Geometry: final body of the model. Coordinates: model frame, mm. Face numbers are marked on the shaded views. A direction names the side the tool comes from. Coordinates: 2 decimals unless noted, no trailing zeros. Write each loop counter-clockwise with the first axis right and the second up, starting at its lowest first coordinate (ties: lowest second). Pieces come first, ordered by that corner, then holes.
from build123d import *

# Parameters (mm, degrees)
BOSS_EXTRUDE1_DEPTH = 6.35
CUT_EXTRUDE1_DEPTH  = 76.2
FILLET1_R           = 12.700000000000001


with BuildPart() as part:
    # Sketch1 → Boss-Extrude1 (new, symmetric)
    with BuildSketch(Plane.XY):
        Polygon((-50.8, 87.98818102450007), (0, 0), (50.79999999999998, 87.98818102450008), (50.800000000000004, -76.19999999999999), (-50.79999999999999, -76.20000000000002), align=None)
    extrude(amount=BOSS_EXTRUDE1_DEPTH, both=True)

    # Sketch2 → Cut-Extrude1 (cut)
    with BuildSketch(Plane(origin=(-50.80000000000058, 87.98818102449974, 0), x_dir=(0, 0, -1), z_dir=(-0.500000000000001, 0.866025403784438, 0))):
        Polygon((3.175000000000003, 0), (-3.1749999999999967, 0), (-3.1749999999999967, 6.35), (3.65e-15, 9.524999999999999), (3.1749999999999994, 6.35), align=None)
    cut_extrude1 = extrude(amount=-CUT_EXTRUDE1_DEPTH, mode=Mode.SUBTRACT)

    # Mirror5: Cut-Extrude1 across plane
    add(cut_extrude1.mirror(Plane(origin=(0, 0, 0), x_dir=(0, 0, 1), z_dir=(1, 0, 0))), mode=Mode.SUBTRACT)

    # Fillet1
    fillet1_edges = [part.edges().sort_by_distance(p)[0] for p in [
        (50.79999999999998, 87.98818102450008, 4.762499999999998),
        (-50.8, 87.98818102450007, -4.762500000000001),
    ]]
    fillet(fillet1_edges, radius=FILLET1_R)


solid = part.part
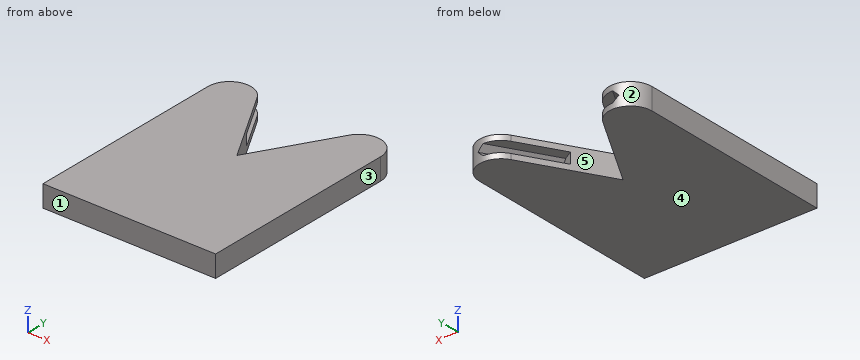
Item 1: Section C-C, the plane x = 32.5. Output: boundary loops of the cut face in (y, z) (3 decimals).
Derived:
outline: (-76.2, -6.35) - (51.99, -6.35) - (51.99, -3.175) - (43.592, -3.175) - (37.242, 0) - (43.592, 3.175) - (51.99, 3.175) - (51.99, 6.35) - (-76.2, 6.35) - close
Item 2: Set-up query: the marked faces 4 and 5. Return all of +Z, -Z, +X, -X, +Y, -Y with unobstructed straight access to the full face (end or side cutting, diameter ignored); none if empty.
Derived:
face 4: -Z, +X, -X, +Y, -Y
face 5: +Z, -Z, +Y
Item 3: Material intervals for probe 1 along Z at (x, y) = (30, 47) (3 decimals); probe 2 along X at (y, z) = (31.5, -5); probe 3 along X at (y, z) = (45, 3), sorted ascending.
Derived:
probe 1: z = -6.35 to -3.175, 3.175 to 6.35
probe 2: x = -50.8 to -18.19, 18.19 to 50.8
probe 3: x = -50.01 to -33.52, 33.52 to 50.01
Item 4: Pull-direction query (X, two-part tool) for the marked faces 1, 2 and 3; classes: released by +X, released by -X, zero draft, split by the parting line, or undercut.
Derived:
face 1: zero draft
face 2: undercut
face 3: released by +X
Item 5: Pin query (flat end, axial travel): pin 1 (1 mm diameter, centred on x = 6.5, z = 3.5, fed in from +Y). Return the tip coordinate at first contact, or that it passes through.
Derived:
pin 1: stops at y = 12.12
Item 6: Section B-B, the plane z = 1.5. Output: boundary loops of the cut face in (x, y), plus the area to 3 significant figures.
Derived:
outline: (-50.8, -76.2) - (50.8, -76.2) - (50.8, 40.59) arc R12.7 ccw to (39.96, 53.15) - (19.65, 17.98) - (12.7, 22) - (0, 0) - (-12.7, 22) - (-19.65, 17.98) - (-39.96, 53.15) arc R12.7 ccw to (-50.8, 40.59) - close
area: 10,800 mm2
Item 7: Section A-A, the plane y = 10. Output: boundary loops of the cut face in (x, z).
Derived:
outline: (-50.8, -6.35) - (-5.77, -6.35) - (-5.77, 6.35) - (-50.8, 6.35) - close; (5.77, -6.35) - (50.8, -6.35) - (50.8, 6.35) - (5.77, 6.35) - close
